Check sheet for the modelled part. Datum: model origin and axes. Units: mm. A direction names the side the tool comes from. Give positions to 0.01 mm unless a question says otherwise; leave off trailing zeros. Write each loop counter-clockwise with the first axis right and the second up, starting at its lowest first coordinate (ties: lowest second). Pieces come first, ordered by that corner, then holes. Notation, with made-up numbers: M 75,27.5 L 123,27.5 A26 ccw 123,55.5 Z; hole C 70.5,59.25 d3. An arc over 180 degrees is marked long. One line per item, written item: value. Start each with the question number.
from build123d import *

# Parameters (mm, degrees)
F1_DEPTH = 20
F2_DEPTH = 12
F3_SIZE  = 2


with BuildPart() as f1:
    # F0 (on Top) → F1 (new body)
    with BuildSketch(Plane.XY):
        with BuildLine():
            Line((-65, 0), (-5, 0))
            ThreePointArc((-5, 0), (-1.464466, 1.464466), (0, 5))
            Line((0, 5), (0, 35))
            ThreePointArc((0, 35), (-1.464466, 38.535534), (-5, 40))
            Line((-5, 40), (-65, 40))
            ThreePointArc((-65, 40), (-68.535534, 38.535534), (-70, 35))
            Line((-70, 35), (-70, 5))
            ThreePointArc((-70, 5), (-68.535534, 1.464466), (-65, 0))
        make_face()
        with BuildLine():
            ThreePointArc((-57, 20), (-55.828427, 22.828427), (-53, 24))
            Line((-53, 24), (-17, 24))
            ThreePointArc((-17, 24), (-14.171573, 22.828427), (-13, 20))
            ThreePointArc((-13, 20), (-14.171573, 17.171573), (-17, 16))
            Line((-17, 16), (-53, 16))
            ThreePointArc((-53, 16), (-55.828427, 17.171573), (-57, 20))
        make_face(mode=Mode.SUBTRACT)
    extrude(amount=F1_DEPTH)

    # F0 (on Top) → F2 (join)
    with BuildSketch(Plane.XY):
        with BuildLine():
            Line((-17, 24), (-53, 24))
            ThreePointArc((-53, 24), (-55.828427, 22.828427), (-57, 20))
            ThreePointArc((-57, 20), (-55.828427, 17.171573), (-53, 16))
            Line((-53, 16), (-17, 16))
            ThreePointArc((-17, 16), (-14.171573, 17.171573), (-13, 20))
            ThreePointArc((-13, 20), (-14.171573, 22.828427), (-17, 24))
        make_face()
    extrude(amount=F2_DEPTH)

    # F3
    f3_edges = [f1.edges().sort_by_distance(p)[0] for p in [
        (-35, 24, 20),
        (-35, 0, 20),
    ]]
    chamfer(f3_edges, length=F3_SIZE)


solid = f1.part
1) Cross-section at A-A (z = 15.25). Record the boundary of the cut face in (x, y).
2) Material ranges on L1, parallel to Y at x = -24, z = 17; L2, parallel to Z at x = -29, y = 20; L3, parallel to X at y = 19, z = 19, recorded low to high. Write a range as from..to.
3) Draft check along X on faces 3 (the flat face through (-1, 20, 19)), 4 (the conical face through (-67.63, 37.69, 19.24)), 5 (the flat face through (-35, 24, 15)). Enter one of: released by +X, released by -X, zero draft, split by the parting line, or undercut.
4) Tool access check on faces 1 (the flat face through (-70, 20, 9)), 2 (the flat face through (-35, 25, 19)). Record the directions out of +Z, -Z, +X, -X, +Y, -Y that give a thin tool (end or side, any length) a straight path to the whole face; none if there is none.
5) Gauge pin test, flat ends, axial feed: pin 1 (4 mm diameter, centred on x = -40, y = 20.5, fed in from +Z); pin 2 (3 mm diameter, centred on x = -22, y = 10.5, fed in from -Z). Record the tip position at first contact, or that the pin passes through.
6) Cross-section at B-B (x = -34.5). Record the boundary of the cut face in (y, z), plus the area to 3 significant figures.
Data:
1. outline: M -70,5 A5 ccw -65,0 L -5,0 A5 ccw 0,5 L 0,35 A5 ccw -5,40 L -65,40 A5 ccw -70,35 Z; hole M -53,16 L -17,16 A4 ccw -17,24 L -53,24 A4 ccw Z
2. L1: y = 0..16, 24..40
2. L2: z = 0..12
2. L3: x = -69..-57.9, -12.1..-1
3. face 3: released by +X
3. face 4: released by -X
3. face 5: undercut
4. face 1: +Z, -Z, -X, +Y, -Y
4. face 2: +Z
5. pin 1: stops at z = 12
5. pin 2: stops at z = 0
6. outline: M 0,0 L 40,0 L 40,18 L 38,20 L 26,20 L 24,18 L 24,12 L 16,12 L 16,18 L 14,20 L 2,20 L 0,18 Z
6. area: 728 mm2
